Input: part model. Units: mm. Frame: model coordinates. Face numbers are marked on the shaded views. Coordinates: 2 decimals unless noted, no trailing zeros. Order: outer loops, then holes, each group sorted by start corner. A loop starts at its lowest first (then second) coordinate and runs counter-clockwise, first axis right, second up. Notation, with made-up numbers: (55, -20.5) -> (66, -20.5) arc R30 cw to (66, 6.5) -> close; hole circle Ø3 at (-14.5, -31.5). An arc over 180 degrees is marked (long way). One line per item, written item: value. Start each with the question number.
from build123d import *

# Parameters (mm, degrees)
SKETCH1_R           = 5
BOSS_EXTRUDE1_DEPTH = 2
SKETCH2_R           = 6
BOSS_EXTRUDE2_DEPTH = 2
SKETCH4_R           = 4
BOSS_EXTRUDE3_DEPTH = 1


with BuildPart() as part:
    # Sketch1 → Boss-Extrude1 (new body)
    with BuildSketch(Plane.XY):
        with BuildLine():
            Line((26.754759572, 15.066584336), (-7.828159274, 35.03304384))
            Line((-7.828159274, 35.03304384), (-3.776725793, 42.017662227))
            Line((-3.776725793, 42.017662227), (-5.864916731, 43.223279828))
            ThreePointArc((-5.864916731, 43.223279828), (-10.564626295, 45.070633496), (-15.599655414, 45.455948092))
            ThreePointArc((-15.599655414, 45.455948092), (-17.660328687, 45.178385552), (-19.671702879, 44.651328476))
            ThreePointArc((-19.671702879, 44.651328476), (-28.5, 40.703193978), (-36.333333333, 35.031731647))
            ThreePointArc((-36.333333333, 35.031731647), (-37.795465247, 33.553359039), (-39.066178094, 31.907544906))
            ThreePointArc((-39.066178094, 31.907544906), (-41.250000425, 27.354424482), (-42, 22.360679775))
            Line((-42, 22.360679775), (-42, 19.950798463))
            Line((-42, 19.950798463), (-33.9254247, 19.967136312))
            Line((-33.9254247, 19.967136312), (-33.9254247, -19.965779701))
            Line((-33.9254247, -19.965779701), (-42, -19.949444575))
            Line((-42, -19.949444575), (-42, -22.360679775))
            ThreePointArc((-42, -22.360679775), (-41.250000425, -27.354424482), (-39.066178094, -31.907544906))
            ThreePointArc((-39.066178094, -31.907544906), (-37.795465247, -33.553359039), (-36.333333333, -35.031731647))
            ThreePointArc((-36.333333333, -35.031731647), (-28.5, -40.703193978), (-19.671702879, -44.651328476))
            ThreePointArc((-19.671702879, -44.651328476), (-17.660328687, -45.178385552), (-15.599655414, -45.455948092))
            ThreePointArc((-15.599655414, -45.455948092), (-10.564626295, -45.070633496), (-5.864916731, -43.223279828))
            Line((-5.864916731, -43.223279828), (-3.808380011, -42.035937798))
            Line((-3.808380011, -42.035937798), (-7.811356047, -35.023340495))
            Line((-7.811356047, -35.023340495), (26.735608761, -15.07764306))
            Line((26.735608761, -15.07764306), (30.807203868, -22.050621128))
            Line((30.807203868, -22.050621128), (32.864916731, -20.862600053))
            ThreePointArc((32.864916731, -20.862600053), (36.81462672, -17.716209014), (39.665833508, -13.548403186))
            ThreePointArc((39.665833508, -13.548403186), (40.455793934, -11.625026513), (41.005036212, -9.619596828))
            ThreePointArc((41.005036212, -9.619596828), (42, 0), (41.005036212, 9.619596828))
            ThreePointArc((41.005036212, 9.619596828), (40.455793934, 11.625026513), (39.665833508, 13.548403186))
            ThreePointArc((39.665833508, 13.548403186), (36.81462672, 17.716209014), (32.864916731, 20.862600053))
            Line((32.864916731, 20.862600053), (30.777898295, 22.067540709))
            Line((30.777898295, 22.067540709), (26.754759572, 15.066584336))
        make_face()
        with Locations((-25, 34.641016151)):
            Circle(SKETCH1_R, mode=Mode.SUBTRACT)
        with Locations((35, 0)):
            Circle(SKETCH1_R, mode=Mode.SUBTRACT)
        with Locations((-25, -34.641016151)):
            Circle(SKETCH1_R, mode=Mode.SUBTRACT)
    extrude(amount=BOSS_EXTRUDE1_DEPTH)

    # Sketch2 → Boss-Extrude2 (add)
    with BuildSketch(Plane.XY.offset(2)):
        with Locations((-25, 34.641016151)):
            Circle(SKETCH2_R)
        with Locations((-25, -34.641016151)):
            Circle(SKETCH2_R)
        with Locations((35, 0)):
            Circle(SKETCH2_R)
    extrude(amount=-BOSS_EXTRUDE2_DEPTH)

    # Sketch4 → Boss-Extrude3 (add)
    with BuildSketch(Plane(origin=(0, 0, 0), x_dir=(-1, 0, 0), z_dir=(0, 0, -1))):
        with Locations(Location((25, 34.641016151, 0), (0, 0, 180))):
            Circle(SKETCH4_R)
        with Locations(Location((-35, 0, 0), (0, 0, 180))):
            Circle(SKETCH4_R)
        with Locations(Location((25, -34.641016151, 0), (0, 0, 180))):
            Circle(SKETCH4_R)
    extrude(amount=BOSS_EXTRUDE3_DEPTH)


solid = part.part
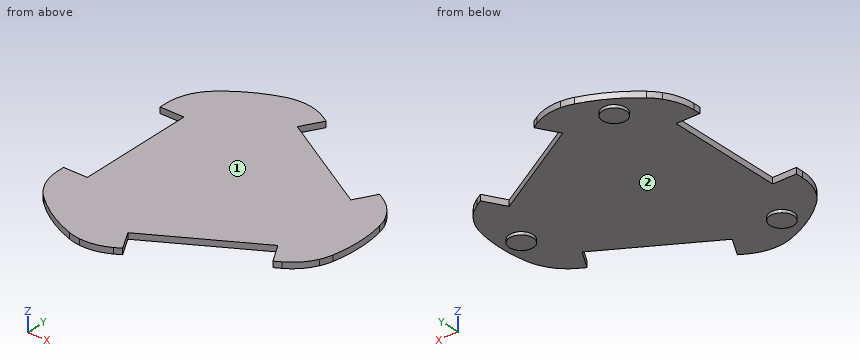
1) Section query D-D, the plane x = -25. Return the cut outline in (y, z).
2) Section query C-C, the plane x = 35. Return the cut outline in (y, z), plus the area to 3 significant figures.
3) Section query A-A, the plane y = 0. Return the cut outline in (x, z), plus the area to 3 significant figures.
4) Pin query (flat end, axial travel): pin 1 Ø1.5 at (x, z) = (4.5, -0.5) entering from -Y; pin 2 Ø25 at (x, y) = (-5, 17.5) entering from -Z; pin 3 Ø0.6 at (y, z) = (-2, 1) entering from -X. Return the tip coordinate at first contact, or that it passes through.
5) Ray query, line 1 along Z through (x, y) = (16.5, 1); line 2 along X through (y, z) = (-13.5, 1.6); line 3 along Y through (x, z) = (-9, 1.1). Return the intervals inside material, ascending. Write a range as from..to.
6) Mould query, pull axis Y, two halves, no side actions, for the marked faces 1 and 2. Classes: +Y half, -Y half, draft (parallel to the pull), parting line (faces both ways), or undercut.
7) Section query B-B, the plane z = 1. Return the cut outline in (x, y).
Entries:
1. outline: (-42.53, 0) -> (-38.64, 0) -> (-38.64, -1) -> (-30.64, -1) -> (-30.64, 0) -> (30.64, 0) -> (30.64, -1) -> (38.64, -1) -> (38.64, 0) -> (42.53, 0) -> (42.53, 2) -> (-42.53, 2) -> close
2. outline: (-19.4, 0) -> (-4, 0) -> (-4, -1) -> (4, -1) -> (4, 0) -> (19.4, 0) -> (19.4, 2) -> (-19.4, 2) -> close
2. area: 85.6 mm2
3. outline: (-33.93, 0) -> (31, 0) -> (31, -1) -> (39, -1) -> (39, 0) -> (42, 0) -> (42, 2) -> (-33.93, 2) -> close
3. area: 160 mm2
4. pin 1: stops at y = -28.24
4. pin 2: stops at z = 0
4. pin 3: stops at x = -33.93
5. line 1: z = 0..2
5. line 2: x = -33.93..39.69
5. line 3: y = -44.63..44.63
6. face 1: draft
6. face 2: undercut
7. outline: (-42, -22.36) arc R17 ccw to (-36.33, -35.03) arc R47 ccw to (-19.67, -44.65) arc R17 ccw to (-5.86, -43.22) -> (-3.81, -42.04) -> (-7.81, -35.02) -> (26.74, -15.08) -> (30.81, -22.05) -> (32.86, -20.86) arc R17 ccw to (41.01, -9.62) arc R47 ccw to (41.01, 9.62) arc R17 ccw to (32.86, 20.86) -> (30.78, 22.07) -> (26.75, 15.07) -> (-7.83, 35.03) -> (-3.78, 42.02) -> (-5.86, 43.22) arc R17 ccw to (-19.67, 44.65) arc R47 ccw to (-36.33, 35.03) arc R17 ccw to (-42, 22.36) -> (-42, 19.95) -> (-33.93, 19.97) -> (-33.93, -19.97) -> (-42, -19.95) -> close
